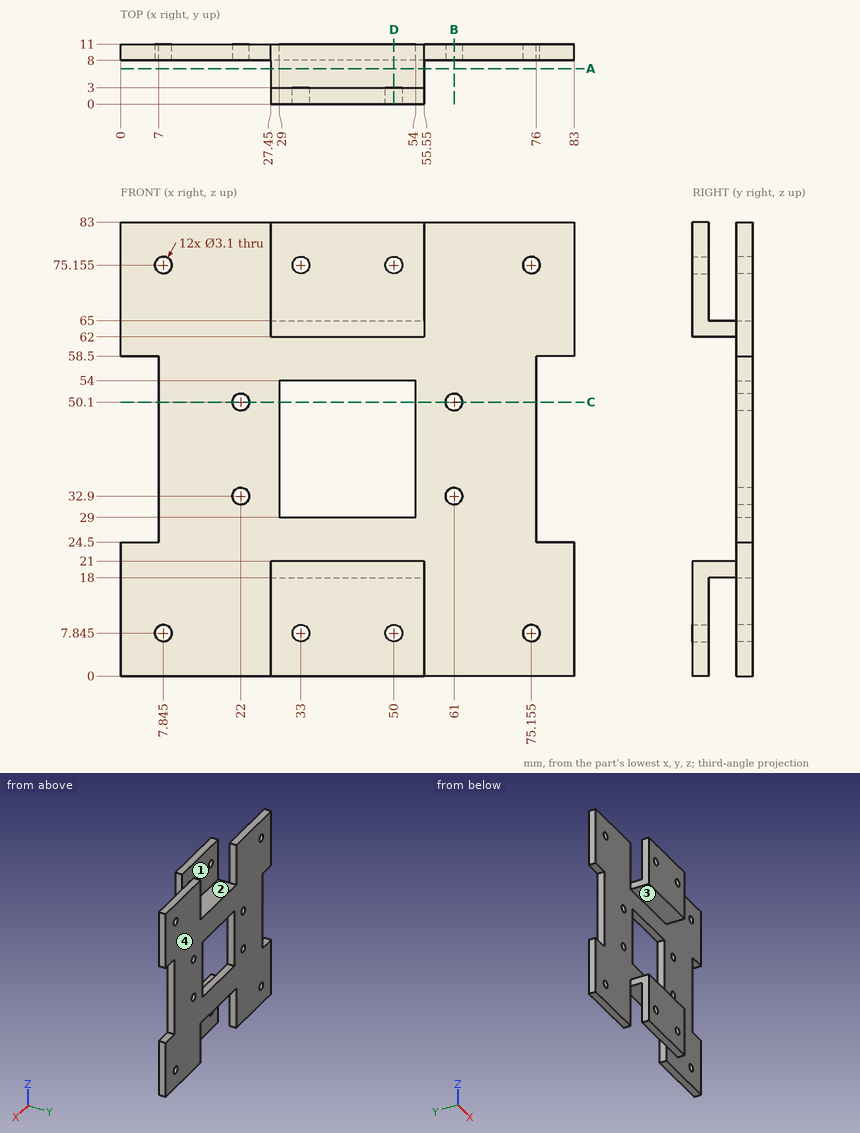
Job drawing, mm, ordinate dimensions from the low corner. One solid piece. A direction names the side the tool comes from. Coordinates: 2 decimals unless noted, no trailing zeros. Loops run counter-clockwise (first coordinate to the right, second up) from the corner with the lowest first, then second, coordinate; pieces in that order, holes last. Notation, with made-up numbers: (-24.5, 25.25) - (-18.5, 25.25) arc R16 ccw to (-18.5, 46.25) - close; hole circle Ø5 at (-20.75, 2.25). An arc over 180 degrees is marked (long way). Write item = value, one per line. Start each with the question number.
Q1. Pull direction X, two halves, no side cores. Call the marked faces 1 and 2: pulls with the +X half, pulls with the -X half, needs draft (parallel to the pull), parting line crosses it, or undercut.
Q2. Cut at C-C, the plane z = 50.1. List the corners of the cut face in (x, y), then the cut area to 3 significant figures.
Q3. Cut at B-B, the plane x = 61. List the corners of the cut face in (y, z).
Q4. Which spindle directions (+Z, -Z, +X, -X, +Y, -Y) get a long thin tool onto all of the face, cutting with end or side? Do the marked faces 3 and 4. Say none if no direction does.
Q5. Cut at D-D, the plane x = 50. List the corners of the cut face in (y, z) (3 decimals), then the cut area to 3 significant figures.
Q6. Drill centre lines: L1, parallel to X at y = 9.5, z = 50.1; L2, parallel to Z at x = 50, y = 2 (3 decimals); L3, parallel to Z at x = 61, y = 10.2. Where is each one in solid material? Low to high.
Q7. Flat gauge pins, fed straight in: pin 1 Ø0.9 at (y, z) = (9.5, 34.5) entering from +X; pin 2 Ø4 at (x, y) = (44.5, 9) entering from +Z; pin 3 Ø14.5 at (x, z) = (38, 10) entering from +Y; pin 4 Ø1.9 at (x, z) = (22, 50.1) entering from +Y. Where does each tip first touch, or does it go through?
Q8. Cut at A-A, the plane y = 6.5. List the corners of the cut face in (x, z).
Computed:
q1.face_1 = needs draft
q1.face_2 = undercut
q2.outline = (7, 8) - (20.45, 8) - (20.45, 11) - (7, 11) - close; (23.55, 8) - (29, 8) - (29, 11) - (23.55, 11) - close; (54, 8) - (59.45, 8) - (59.45, 11) - (54, 11) - close; (62.55, 8) - (76, 8) - (76, 11) - (62.55, 11) - close
q2.area = 113 mm²
q3.outline = (8, 0) - (11, 0) - (11, 31.35) - (8, 31.35) - close; (8, 34.45) - (11, 34.45) - (11, 48.55) - (8, 48.55) - close; (8, 51.65) - (11, 51.65) - (11, 83) - (8, 83) - close
q4.face_3 = +X, -X, -Y
q4.face_4 = +Z, -Z, +X, -X, +Y
q5.outline = (0, 0) - (3, 0) - (3, 6.295) - (0, 6.295) - close; (0, 9.395) - (3, 9.395) - (3, 18) - (11, 18) - (11, 29) - (8, 29) - (8, 21) - (0, 21) - close; (0, 62) - (8, 62) - (8, 54) - (11, 54) - (11, 65) - (3, 65) - (3, 73.605) - (0, 73.605) - close; (0, 76.705) - (3, 76.705) - (3, 83) - (0, 83) - close
q5.area = 203 mm²
q6.L1 = 7 to 20.45, 23.55 to 29, 54 to 59.45, 62.55 to 76
q6.L2 = 0 to 6.295, 9.395 to 21, 62 to 73.605, 76.705 to 83
q6.L3 = 0 to 31.35, 34.45 to 48.55, 51.65 to 83
q7.pin_1 = 76
q7.pin_2 = 65
q7.pin_3 = 3
q7.pin_4 = through
q8.outline = (27.45, 18) - (55.55, 18) - (55.55, 21) - (27.45, 21) - close; (27.45, 62) - (55.55, 62) - (55.55, 65) - (27.45, 65) - close
